```python
from build123d import *

# Parameters (mm, degrees)
SKETCH1_W                 = 95.9
SKETCH1_H                 = 93.2
SKETCH1_R                 = 2
SKETCH1_W_2               = 70
SKETCH1_H_2               = 70
BOSS_EXTRUDE1_DEPTH       = 1.58
SKETCH2_R                 = 2.5
BOSS_EXTRUDE2_DEPTH       = 6
M3X0_5_TAPPED_HOLE2_D     = 2.5
M3X0_5_TAPPED_HOLE2_DEPTH = 6
M3X0_5_TAPPED_HOLE2_TIP   = 0.751075774


with BuildPart() as part:
    # Sketch1 → Boss-Extrude1 (new body)
    with BuildSketch(Plane(origin=(0, 0, 0), x_dir=(1, 0, 0), z_dir=(0, 1, 0))):
        Rectangle(SKETCH1_W, SKETCH1_H)
        with Locations((0, 39.1)):
            Circle(SKETCH1_R, mode=Mode.SUBTRACT)
        with Locations((41.95, 0)):
            Circle(SKETCH1_R, mode=Mode.SUBTRACT)
        with Locations((0, -39.1)):
            Circle(SKETCH1_R, mode=Mode.SUBTRACT)
        with Locations((-41.95, 0)):
            Circle(SKETCH1_R, mode=Mode.SUBTRACT)
        Rectangle(SKETCH1_W_2, SKETCH1_H_2, mode=Mode.SUBTRACT)
    extrude(amount=BOSS_EXTRUDE1_DEPTH)

    # Sketch2 → Boss-Extrude2 (add)
    with BuildSketch(Plane(origin=(0, 1.58, 0), x_dir=(1, 0, 0), z_dir=(0, 1, 0))):
        with Locations((37.355, 42.8635)):
            Circle(SKETCH2_R)
        with Locations((-36.325, 42.8625)):
            Circle(SKETCH2_R)
        with Locations((-38.865, -42.8625)):
            Circle(SKETCH2_R)
        with Locations((41.145, -42.8625)):
            Circle(SKETCH2_R)
    extrude(amount=BOSS_EXTRUDE2_DEPTH)

    # M3x0.5 Tapped Hole2
    with Locations(Plane(origin=(-36.325, 7.58, -42.8625), x_dir=(0, 0, 1), z_dir=(0, 1, 0))):
        with Locations((0, 0), (85.725, -2.54), (85.725, 77.47), (-0.001, 73.68)):
            Hole(M3X0_5_TAPPED_HOLE2_D / 2, depth=M3X0_5_TAPPED_HOLE2_DEPTH)
            with Locations((0, 0, -(M3X0_5_TAPPED_HOLE2_DEPTH + M3X0_5_TAPPED_HOLE2_TIP / 2))):  # 118° drill point
                Cone(0, M3X0_5_TAPPED_HOLE2_D / 2, M3X0_5_TAPPED_HOLE2_TIP, mode=Mode.SUBTRACT)


solid = part.part
```
Can you work these out from the model? Positions are in its coordinate system, mm. A direction names the side the tool comes from. Coordinates: 2 decimals unless noted, no trailing zeros. Write each loop counter-clockwise with the first axis right and the second up, starting at its lowest first coordinate (ties: lowest second). Pieces come first, ordered by that corner, then holes. Notation, with made-up numbers: (77, 4) - (106, 4) arc R24 cw to (106, 26) - close; hole circle Ø9 at (85, -13). An arc over 180 degrees is marked (long way). Return JSON: item names as keys, results as strings.
Q1. If we section it at C-C (z = 17): Please give me the cut outline in (x, y).
Computed values:
{"outline": "(-47.95, 0) - (-35, 0) - (-35, 1.58) - (-47.95, 1.58) - close; (35, 0) - (47.95, 0) - (47.95, 1.58) - (35, 1.58) - close"}
Q2. I'm going to push flat-ended pins straight in: pin 1 Ø4 at (x, y) = (-37.5, 2.5) entering from +Z; pin 2 Ø2 at (x, z) = (-38.86, 42.86) entering from +Y; pin 3 Ø2.5 at (x, z) = (41.95, 0) entering from +Y; pin 4 Ø6.5 at (x, z) = (0, -39.1) entering from +Y. Where does each tip first touch, or does it pass through?
Computed values:
{"pin 1": "stops at z = 46.6", "pin 2": "stops at y = 1.43", "pin 3": "passes through", "pin 4": "stops at y = 1.58"}
Q3. If we section it at A-A (z = 0): Please give me the cut outline in (x, y).
Computed values:
{"outline": "(-47.95, 0) - (-43.95, 0) - (-43.95, 1.58) - (-47.95, 1.58) - close; (-39.95, 0) - (-35, 0) - (-35, 1.58) - (-39.95, 1.58) - close; (35, 0) - (39.95, 0) - (39.95, 1.58) - (35, 1.58) - close; (43.95, 0) - (47.95, 0) - (47.95, 1.58) - (43.95, 1.58) - close"}
Q4. Please list where these lines run through material, in increasing order: L1, parallel to Z at x = -37, y = 4; L2, parallel to Z at x = -5, y = 1.5; L3, parallel to X at y = 1.15, z = -39.1. Write a range as from..to.
Computed values:
{"L1": "z = -45.27..-43.91, -41.81..-40.46, 41.2..44.53", "L2": "z = -46.6..-35, 35..46.6", "L3": "x = -47.95..-2, 2..47.95"}
Q5. If we section it at B-B (x = -19.5): Please give me the cut outline in (y, z).
Computed values:
{"outline": "(0, -46.6) - (1.58, -46.6) - (1.58, -35) - (0, -35) - close; (0, 35) - (1.58, 35) - (1.58, 46.6) - (0, 46.6) - close"}
Q6. Thinking about a two-plate mould opening in X: for faces 1 (the cylindrical face through (-36.48, 4.54, 42.11)), 2 (the flat face through (-36, 0, -4)), which applies, +X half, -X half, draft (parallel to the pull), parting line (faces both ways), or undercut?
Computed values:
{"face 1": "undercut", "face 2": "draft"}
Q7. On a 3-axis mill with a long thin cutter (end or side, diameter ignored), from which of +Z, -Z, +X, -X, +Y, -Y can I reach the whole of each face in a straight line? I mean faces 3 (the flat face through (-35, 7.58, -42)), 4 (the cylindrical face through (37.41, 4.538, -41.615)). Say none if no direction works.
Computed values:
{"face 3": "+Z, -Z, +X, -X, +Y", "face 4": "+Y"}
Q8. If we section it at D-D (y = 5.5): Count the separate pieces of the cut face and the enclosed holes in it, then the cut area to 3 significant figures.
Computed values:
{"separate pieces": "4", "enclosed holes": "4", "area": "58.9 mm2"}
